Part model, mm, in its own coordinate system. Give positions to 0.01 mm unless a question says otherwise; leave off trailing zeros. Write each loop counter-clockwise with the first axis right and the second up, starting at its lowest first coordinate (ties: lowest second). Pieces come first, ordered by that corner, then holes. Notation, with made-up numbers: M 68,55.5 L 82,55.5 A12 cw 82,73.5 Z; hole C -11,38 d10. An arc over 180 degrees is marked long. Answer as CSV lines item,"result". Start each with the question number.
1) Slice it at D-D, the plane x = 35. Give the cut face in (y, z), plus the area to 3 significant figures.
2) Wall check: line 1 along Z through (x, y) = (-15.5, -1); line 2 along X through (y, z) = (-2.5, -29); line 3 along Z through (x, y) = (-25.5, -6). Give the ranges that are in metal, low to high. Write a range as from..to.
3) Slice it at A-A, the plane x = 0. Give the cut face in (y, z).
4) Slice it at C-C, the plane y = -4.5. Give the number of separate pieces and of enclosed holes in the cut face, plus the area to 3 significant figures.
5) Pin check, flat tip, straight feed: pin 1 Ø3 at (y, z) = (-3, -34) entering from -X. Stop position of the tip, or through.
6) Slice it at B-B, the plane z = -44.45. Give the cut face in (x, y) (3 decimals).
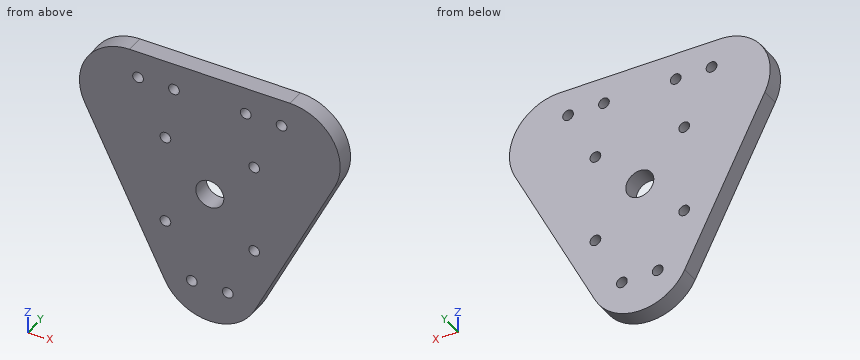
```python
from build123d import *

# Parameters (mm, degrees)
BOSS_EXTRUDE1_DEPTH       = 6.35
F_6_CLEARANCE_HOLE1_D     = 3.7973
FILLET1_R                 = 17.78
F_7_16_20_TAPPED_HOLE1_D  = 9.92124
F_6_CLEARANCE_HOLE2_D     = 3.7973
F_6_CLEARANCE_HOLE2_DEPTH = 6.35


with BuildPart() as part:
    # Sketch1 → Boss-Extrude1 (new body)
    with BuildSketch(Plane(origin=(0, 0, 0), x_dir=(1, 0, 0), z_dir=(0, 1, 0))):
        Polygon((-57.15, 0), (0, 114.3), (57.15, 0), align=None)
    extrude(amount=-BOSS_EXTRUDE1_DEPTH)

    # #6 Clearance Hole1 (through all)
    with Locations(Plane(origin=(0, 0, 0), x_dir=(1, 0, 0), z_dir=(0, 1, 0))):
        with Locations((25.4, 9.525), (12.7, 9.525), (-6.35, 79.375), (6.35, 79.375), (-25.4, 9.525), (-12.7, 9.525)):
            Hole(F_6_CLEARANCE_HOLE1_D / 2)

    # Fillet1
    fillet1_edges = [part.edges().sort_by_distance(p)[0] for p in [
        (-57.15, -3.175, 0),
        (0, -3.175, -114.3),
        (57.15, -3.175, 0),
    ]]
    fillet(fillet1_edges, radius=FILLET1_R)

    # 7/16-20 Tapped Hole1 (through all)
    with Locations(Plane(origin=(0, 0, 0), x_dir=(1, 0, 0), z_dir=(0, 1, 0))):
        with Locations((0, 44.45)):
            Hole(F_7_16_20_TAPPED_HOLE1_D / 2)

    # #6 Clearance Hole2
    with Locations(Plane(origin=(0, 0, 0), x_dir=(1, 0, 0), z_dir=(0, 1, 0))):
        with Locations((-15.715448212, 60.165448212), (15.715448212, 28.734551788), (-15.715448212, 28.734551788), (15.715448212, 60.165448212)):
            Hole(F_6_CLEARANCE_HOLE2_D / 2, depth=F_6_CLEARANCE_HOLE2_DEPTH)


solid = part.part
```
Found:
1,outline,"M -6.35,-44.3 L 0,-44.3 L 0,-1.28 L -6.35,-1.28 Z"
1,area,"273 mm²"
2,line 1,"-83.25..-62.05, -58.28..-30.62, -26.85..0"
2,line 2,"-42.65..-17.6, -13.84..13.84, 17.6..42.65"
2,line 3,"-63.3..-11.42, -7.63..0"
3,outline,"M -6.35,-92.32 L 0,-92.32 L 0,-49.41 L -6.35,-49.41 Z; M -6.35,-39.49 L 0,-39.49 L 0,0 L -6.35,0 Z"
4,separate pieces,"1"
4,enclosed holes,"11"
4,area,"5,680 mm²"
5,pin 1,"x = -40.9"
6,outline,"M -34.925,-6.35 L -4.961,-6.35 L -4.961,0 L -34.925,0 Z; M 4.961,-6.35 L 34.925,-6.35 L 34.925,0 L 4.961,0 Z"
